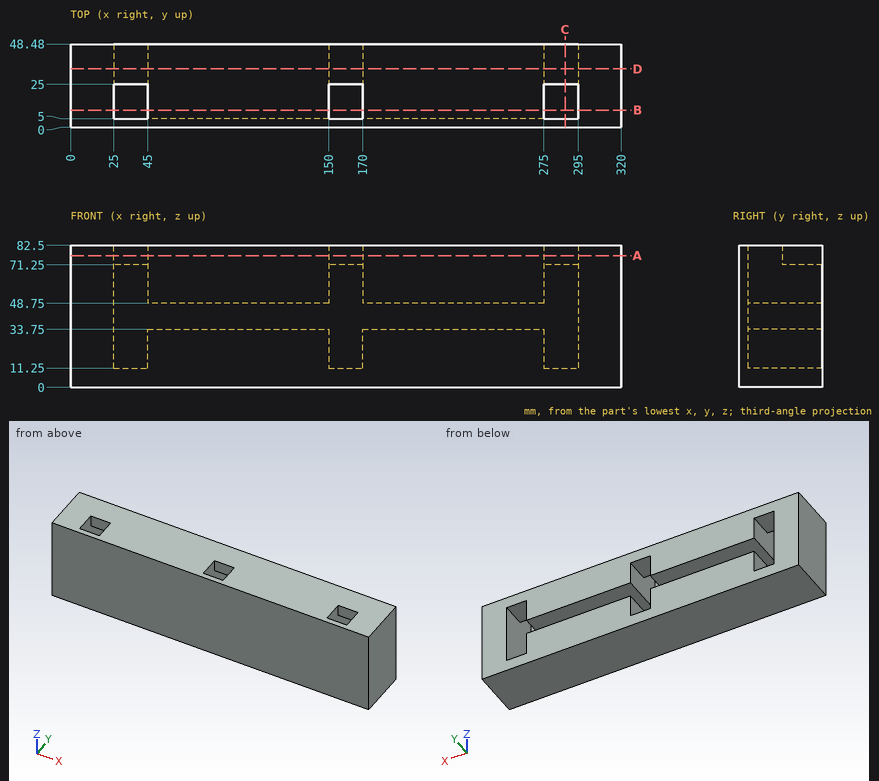
Design review of the part shown in the three views and the two pictorial views. Dimensions are in mm from the part's minimum x, y and z. Round coordinates to 2 decimals unless told otherwise and drop trailing zeros. Loops run counter-clockwise (first coordinate to the right, second up) from the corner with the lowest first, then second, coordinate; pieces in that order, holes last.
1) Consider section A-A on z = 76.5. State the section outline as (x, y) points.
Values follow:
outline: (0, 0) - (320, 0) - (320, 48.48) - (0, 48.48) - close; hole (25, 5) - (45, 5) - (45, 25) - (25, 25) - close; hole (150, 5) - (170, 5) - (170, 25) - (150, 25) - close; hole (275, 5) - (295, 5) - (295, 25) - (275, 25) - close
2) Consider section D-D on y = 34. State the section outline as (x, z) points, then the cut area to 4 significant figures.
Values follow:
outline: (0, 0) - (320, 0) - (320, 82.5) - (0, 82.5) - close; hole (25, 11.25) - (45, 11.25) - (45, 33.75) - (150, 33.75) - (150, 11.25) - (170, 11.25) - (170, 33.75) - (275, 33.75) - (275, 11.25) - (295, 11.25) - (295, 71.25) - (275, 71.25) - (275, 48.75) - (170, 48.75) - (170, 71.25) - (150, 71.25) - (150, 48.75) - (45, 48.75) - (45, 71.25) - (25, 71.25) - close
area: 19,650 mm2
3) Consider section B-B on y = 10. State the section outline as (x, z) points, then the cut area to 3 significant figures.
Values follow:
outline: (0, 0) - (320, 0) - (320, 82.5) - (295, 82.5) - (295, 11.25) - (275, 11.25) - (275, 33.75) - (170, 33.75) - (170, 11.25) - (150, 11.25) - (150, 33.75) - (45, 33.75) - (45, 11.25) - (25, 11.25) - (25, 82.5) - (0, 82.5) - close; (45, 48.75) - (150, 48.75) - (150, 82.5) - (45, 82.5) - close; (170, 48.75) - (275, 48.75) - (275, 82.5) - (170, 82.5) - close
area: 19,000 mm2
4) Consider section C-C on x = 287.5. State the section outline as (y, z) points.
Values follow:
outline: (0, 0) - (48.48, 0) - (48.48, 11.25) - (5, 11.25) - (5, 82.5) - (0, 82.5) - close; (25, 71.25) - (48.48, 71.25) - (48.48, 82.5) - (25, 82.5) - close
5) Wall thickness on line 1 along X through (y, z) = (10.5, 49); line 2 along Z through (x, y) = (78.5, 21); line 3 along X through (y, z) = (36, 43): over which ranges is each line inside the solid? List them lowest first.
Values follow:
line 1: x = 0 to 25, 45 to 150, 170 to 275, 295 to 320
line 2: z = 0 to 33.75, 48.75 to 82.5
line 3: x = 0 to 25, 295 to 320
